from build123d import *

# Parameters (mm, degrees)
F1_DEPTH  = 10
F0_R      = 5
F2_DEPTH  = 5
F2_FACE_R = 5
F3_DEPTH  = 10


with BuildPart() as f1:
    # F0 (on Front) → F1 (new body)
    with BuildSketch(Plane.XZ):
        with BuildLine():
            ThreePointArc((8.6602540378, 30), (9.6592582629, 27.588190451), (10, 25))
            ThreePointArc((10, 25), (-2.588190451, 15.3407417371), (-8.6602540378, 30))
            Line((-8.6602540378, 30), (-30.3108891325, -7.5))
            ThreePointArc((-30.3108891325, -7.5), (-19.0624446436, -2.8407417371), (-11.6506350946, -12.5))
            ThreePointArc((-11.6506350946, -12.5), (-14.5795672827, -19.5710678119), (-21.6506350946, -22.5))
            Line((-21.6506350946, -22.5), (21.6506350946, -22.5))
            ThreePointArc((21.6506350946, -22.5), (12.9903810568, -7.5), (30.3108891325, -7.5))
            Line((30.3108891325, -7.5), (8.6602540378, 30))
        make_face()
    extrude(amount=-F1_DEPTH)

    # F0 (on Front) → F2 (join)
    with BuildSketch(Plane.XZ):
        with BuildLine():
            ThreePointArc((-8.6602540378, 30), (-2.588190451, 15.3407417371), (10, 25))
            ThreePointArc((10, 25), (9.6592582629, 27.588190451), (8.6602540378, 30))
            ThreePointArc((8.6602540378, 30), (0, 35), (-8.6602540378, 30))
        make_face()
        with Locations((0, 25)):
            Circle(F0_R, mode=Mode.SUBTRACT)
        with BuildLine():
            ThreePointArc((-11.6506350946, -12.5), (-19.0624446436, -2.8407417371), (-30.3108891325, -7.5))
            ThreePointArc((-30.3108891325, -7.5), (-30.3108891325, -17.5), (-21.6506350946, -22.5))
            ThreePointArc((-21.6506350946, -22.5), (-14.5795672827, -19.5710678119), (-11.6506350946, -12.5))
        make_face()
        with Locations((-21.6506350946, -12.5)):
            Circle(F0_R, mode=Mode.SUBTRACT)
        with BuildLine():
            ThreePointArc((31.6506350946, -12.5), (31.3098933575, -9.911809549), (30.3108891325, -7.5))
            ThreePointArc((30.3108891325, -7.5), (12.9903810568, -7.5), (21.6506350946, -22.5))
            ThreePointArc((21.6506350946, -22.5), (28.7217029065, -19.5710678119), (31.6506350946, -12.5))
        make_face()
        with Locations((21.6506350946, -12.5)):
            Circle(F0_R, mode=Mode.SUBTRACT)
    extrude(amount=F2_DEPTH)

    # F2_face (on face) → F3 (join)
    with BuildSketch(Plane(origin=(0, 0, 25), x_dir=(1, 0, 0), z_dir=(0, 1, 0))):
        with BuildLine():
            ThreePointArc((8.6602540378, -5), (9.6592582629, -2.588190451), (10, 0))
            ThreePointArc((10, 0), (-2.588190451, 9.6592582629), (-8.6602540378, -5))
            ThreePointArc((-8.6602540378, -5), (0, -10), (8.6602540378, -5))
        make_face()
        Circle(F2_FACE_R, mode=Mode.SUBTRACT)
        with BuildLine():
            ThreePointArc((21.6506350946, 47.5), (12.9903810568, 32.5), (30.3108891325, 32.5))
            ThreePointArc((30.3108891325, 32.5), (30.3108891325, 42.5), (21.6506350946, 47.5))
        make_face()
        with Locations((21.6506350946, 37.5)):
            Circle(F2_FACE_R, mode=Mode.SUBTRACT)
        with BuildLine():
            ThreePointArc((-21.6506350946, 47.5), (-30.3108891325, 42.5), (-30.3108891325, 32.5))
            ThreePointArc((-30.3108891325, 32.5), (-12.9903810568, 32.5), (-21.6506350946, 47.5))
        make_face()
        with Locations((-21.6506350946, 37.5)):
            Circle(F2_FACE_R, mode=Mode.SUBTRACT)
    extrude(amount=F3_DEPTH)


solid = f1.part
Input: part model. Units: mm. Frame: model coordinates. A direction names the side the tool comes from. Coordinates: 2 decimals unless noted, no trailing zeros. Loops run counter-clockwise (first coordinate to the right, second up) from the corner with the lowest first, then second, coordinate; pieces in that order, holes last. Notation, with made-up numbers: (87.5, 28.25) - (143.5, 28.25) arc R16 cw to (143.5, 53.25) - close; hole circle Ø8 at (-14.5, 39.5). An arc over 180 degrees is marked (long way). Answer in a Markdown table with one row per item. Add a question column.
Item 1: Section query A-A on y = -0.75. Return the cut outline in (x, z).
Item 2: Access query for faces 5 (the flat face through (0, 0, -2)), 6 (the flat face through (19.637, 4.93, 10.988)). Directions: +Z, -Z, +X, -X, +Y, -Y. A direction counts if a zero-diameter tool reaches every point of the face in a straight line with its end or side. Return the directions, or none.
Item 3: Section query D-D on z = 25. Return the cut outline in (x, y), then the cut area to 3 significant figures.
Item 4: Section query B-B on x = 0. Return the cut outline in (y, z), then the cut area to 3 significant figures.
Item 5: Line query: line 1 along X through (y, z) = (4.25, -12.5); line 2 along X through (y, z) = (-1, 25); line 3 along Y through (x, z) = (0, 3). Output: solid intervals per line, ascending. Write a range as [from, to].
Item 6: Contact query for flat-ended pins moving along their axis: P1, Ø10, axis at x = 22, z = 19, coming from the +Y side; P2, Ø12, axis at x = -24.5, z = 8, coming from the -Y side; P3, Ø8, axis at y = 3.5, z = -3, coming from the +X side; P4, Ø5, axis at x = 5, y = -1, coming from the -Z side. Output: stop coordinate, or through.
Item 7: Section query C-C on y = 4.75. Return the cut outline in (x, z), then the cut area to 3 significant figures.
Item 8: Mould query, pull axis X, two halves, no side actions, for faces 1 (the cylindrical face through (-16.88, 2.39, -14)), 2 (the flat face through (-19.334, 4.93, 11.512)), 3 (the flat face through (0, 5, -22.5)), 4 (the cylindrical face through (-1.08, 2.39, 29.88)). Classes: released by +X, released by -X, zero draft, split by the parting line, or undercut.
Recorded:
| question | item | result |
|---|---|---|
| 1 | outline | circle Ø20 at (-21.65, -12.5); circle Ø20 at (0, 25); circle Ø20 at (21.65, -12.5); hole circle Ø10 at (-21.65, -12.5); hole circle Ø10 at (0, 25); hole circle Ø10 at (21.65, -12.5) |
| 2 | face 5 | -Y |
| 2 | face 6 | +Z, +X, +Y, -Y |
| 3 | outline | (-11.55, 0) - (-10, 0) - (-10, -5) - (-5, -5) - (-5, 10) - (-11.55, 10) - close; (5, -5) - (10, -5) - (10, 0) - (11.55, 0) - (11.55, 10) - (5, 10) - close |
| 3 | area | 181 mm^2 |
| 4 | outline | (-5, 15) - (0, 15) - (0, -22.5) - (10, -22.5) - (10, 20) - (-5, 20) - close; (-5, 30) - (10, 30) - (10, 35) - (-5, 35) - close |
| 4 | area | 525 mm^2 |
| 5 | line 1 | [-31.65, -26.65], [-16.65, 16.65], [26.65, 31.65] |
| 5 | line 2 | [-10, -5], [5, 10] |
| 5 | line 3 | [0, 10] |
| 6 | P1 | through |
| 6 | P2 | y = 0 |
| 6 | P3 | x = 30.02 |
| 6 | P4 | z = -22.5 |
| 7 | outline | (-30.31, -7.5) arc R10 ccw to (-21.65, -22.5) - (21.65, -22.5) arc R10 ccw to (30.31, -7.5) - (8.66, 30) arc R10 ccw to (-8.66, 30) - close; hole circle Ø10 at (-21.65, -12.5); hole circle Ø10 at (0, 25); hole circle Ø10 at (21.65, -12.5) |
| 7 | area | 2,190 mm^2 |
| 8 | face 1 | undercut |
| 8 | face 2 | released by -X |
| 8 | face 3 | zero draft |
| 8 | face 4 | undercut |
